Source: CAD feature listing. Evaluate the final solid. Frame: model axes, mm. A direction names the side the tool comes from. Give positions to 0.01 mm unless a question says otherwise; leave off trailing zeros. Loops run counter-clockwise (first coordinate to the right, second up) from the corner with the lowest first, then second, coordinate; pieces in that order, holes last.
from build123d import *

# Parameters (mm, degrees)
SKETCH1_R           = 12.7
BOSS_EXTRUDE1_DEPTH = 4
SKETCH2_R           = 6.35
BOSS_EXTRUDE2_DEPTH = 16
SKETCH3_R           = 4
CUT_EXTRUDE1_DEPTH  = 27.880848201
SKETCH4_R           = 1.5
CUT_EXTRUDE2_DEPTH  = 25.053689946
CHAMFER1_SIZE       = 1.5


with BuildPart() as part:
    # Sketch1 → Boss-Extrude1 (new body)
    with BuildSketch(Plane.XY):
        Circle(SKETCH1_R)
    extrude(amount=BOSS_EXTRUDE1_DEPTH)

    # Sketch2 → Boss-Extrude2 (add)
    with BuildSketch(Plane.XY.offset(4)):
        Circle(SKETCH2_R)
    extrude(amount=BOSS_EXTRUDE2_DEPTH)

    # Sketch3 → Cut-Extrude1 (cut, through all)
    with BuildSketch(Plane(origin=(0, 0, 0), x_dir=(-1, 0, 0), z_dir=(0, 0, -1))):
        Circle(SKETCH3_R)
    extrude(amount=-CUT_EXTRUDE1_DEPTH, mode=Mode.SUBTRACT)

    # Sketch4 → Cut-Extrude2 (cut, through all)
    with BuildSketch(Plane.XY.offset(4)):
        with Locations((0, 9.679602242)):
            Circle(SKETCH4_R)
        with Locations((8.38278144, -4.839801121)):
            Circle(SKETCH4_R)
        with Locations((-8.38278144, -4.839801121)):
            Circle(SKETCH4_R)
    extrude(amount=-CUT_EXTRUDE2_DEPTH, mode=Mode.SUBTRACT)

    # Chamfer1
    chamfer1_edges = [part.edges().sort_by_distance(p)[0] for p in [
        (-1.5, 9.679602242, 0),
        (6.88278144, -4.839801121, 0),
        (-9.88278144, -4.839801121, 0),
    ]]
    chamfer(chamfer1_edges, length=CHAMFER1_SIZE)


solid = part.part
1) Pull-direction query (Y, two-part tool) for faces 1 (the cylindrical face through (-0.325, 8.215, 2.768)), 2 (the cylindrical face through (-2.75, -12.4, 1.97)), 3 (the flat face through (-3, 3, 0)); classes: released by +Y, released by -Y, zero draft, split by the parting line, or undercut.
Checks:
face 1: undercut
face 2: split by the parting line
face 3: zero draft
2) Cut plane A-A (y = 0). Return loops of the section in (x, z), and give its area (3 significant figures).
Checks:
outline: (-12.7, 0) - (-4, 0) - (-4, 20) - (-6.35, 20) - (-6.35, 4) - (-12.7, 4) - close; (4, 0) - (12.7, 0) - (12.7, 4) - (6.35, 4) - (6.35, 20) - (4, 20) - close
area: 145 mm2
3) Contact query for flat-ended pins moving along their axis: P1, Ø2.5, axis at x = 0, y = 9.68, coming from the +Z side; P2, Ø8, axis at x = -2, z = 9.5, coming from the -Y side; P3, Ø12.5, axis at x = -0.5, y = -2.5, coming from the +Z side; P4, Ø5, axis at x = 2, z = 10, coming from the +Y side. Output: stop coordinate, or through.
Checks:
P1: passes through
P2: stops at y = -6.35
P3: stops at z = 20
P4: stops at y = 6.35
4) Cut plane B-B (x = 0). State how many separate pieces and enclosed holes the cut face has, and give its area (3 significant figures).
Checks:
separate pieces: 3
enclosed holes: 0
area: 131 mm2
5) Ray query, probe 1 along Y at (x, z) = (0, 3.1); probe 2 along Z at (x, y) = (-4, 7.75); probe 3 along Y at (x, z) = (0.5, 2). Return the intervals inside material, ascending.
Checks:
probe 1: y = -12.7 to -4, 4 to 8.18, 11.18 to 12.7
probe 2: z = 0 to 4
probe 3: y = -12.69 to -3.97, 3.97 to 8.27, 11.09 to 12.69
6) Cut plane D-D (z = 2). Return loops of the section in (x, y).
Checks:
outline: circle Ø25.4 at (0, 0); hole circle Ø3 at (-8.38, -4.84); hole circle Ø8 at (0, 0); hole circle Ø3 at (0, 9.68); hole circle Ø3 at (8.38, -4.84)
7) Reachability of faces 4 (the cylindrical face through (9.814, -4.389, 2.768)), 5 (the flat face through (3, 6, 4)) from +Z, -Z, +X, -X, +Y, -Y: full face, straight path, thin tool, end or side. Return the list, or none.
Checks:
face 4: +Z, -Z
face 5: +Z
8) Cut plane C-C (z = 4.5). Return loops of the section in (x, y), and give its area (3 significant figures).
Checks:
outline: circle Ø12.7 at (0, 0); hole circle Ø8 at (0, 0)
area: 76.4 mm2
